from build123d import *

# Parameters (mm, degrees)
SKETCH_W       = 31.75
SKETCH_H       = 31.75
SKETCH_W_2     = 26.2128
SKETCH_H_2     = 26.2128
PAD_DEPTH      = 152.4
PAD_DEPTH_BACK = 152.4
POCKET_DEPTH   = 31.75


with BuildPart() as part:
    # Sketch → Pad (new body, two sides)
    with BuildSketch(Plane.YZ) as pad_sk:
        Rectangle(SKETCH_W, SKETCH_H)
        Rectangle(SKETCH_W_2, SKETCH_H_2, mode=Mode.SUBTRACT)
    extrude(amount=PAD_DEPTH)
    extrude(pad_sk.sketch, amount=-PAD_DEPTH_BACK)

    # Sketch001 → Pocket (cut)
    with BuildSketch(Plane(origin=(0, 0, 15.875), x_dir=(0, -1, 0), z_dir=(0, 0, 1))):
        Polygon((15.875, 152.4), (-15.875, 152.4), (-15.875, 120.65), align=None)
    pocket = extrude(amount=-POCKET_DEPTH, mode=Mode.SUBTRACT)

    # Mirrored: Pocket across Sketch001 H_Axis
    add(pocket.mirror(Plane(origin=(0, 0, 15.875), x_dir=(0, 0, 1), z_dir=(1, 0, 0))), mode=Mode.SUBTRACT)


solid = part.part
Model file for the job. Use its own axes, mm. A direction names the side the tool comes from. Give positions to 0.01 mm unless a question says otherwise; leave off trailing zeros. Order: outer loops, then holes, each group sorted by start corner. A loop starts at its lowest first (then second) coordinate and runs counter-clockwise, first axis right, second up. Notation, with made-up numbers: (33, -36.75) - (60, -36.75) arc R20 cw to (60, -9.75) - close; hole circle Ø4 at (82.25, 54.5). An arc over 180 degrees is marked (long way). One line per item, written item: value.
Item 1: Two-plate mould, pull along Z, no slides. Class faces 3 (the flat face through (2, 0, -15.875)), 4 (the flat face through (136.303, 0.222, -13.889)), 5 (the flat face through (2, 0, -13.106)): released by +Z, released by -Z, zero draft, split by the parting line, or undercut.
Response values:
face 3: released by -Z
face 4: zero draft
face 5: undercut
Item 2: Pin check, flat tips, straight feed: pin 1 Ø10 at (y, z) = (-10, -7) entering from -X (3 decimals); pin 2 Ø6 at (y, z) = (5.5, 12.5) entering from -X; pin 3 Ø8 at (y, z) = (7, -5.5) entering from -X. Stop position of each tip, or through.
Response values:
pin 1: x = -151.525
pin 2: x = -133.96
pin 3: through
Item 3: Slice it at A-A (z = 1). List the corners of the cut face in (x, y) (3 decimals).
Response values:
outline: (-152.4, -15.875) - (152.4, -15.875) - (149.631, -13.106) - (-149.631, -13.106) - close; (-123.419, 13.106) - (123.419, 13.106) - (120.65, 15.875) - (-120.65, 15.875) - close
Item 4: Slice it at D-D (x = -129.5). List the corners of the cut face in (y, z) (3 decimals), then the cut area to 3 significant figures.
Response values:
outline: (-15.875, -15.875) - (7.025, -15.875) - (7.025, -13.106) - (-13.106, -13.106) - (-13.106, 13.106) - (7.025, 13.106) - (7.025, 15.875) - (-15.875, 15.875) - close
area: 199 mm2
Item 5: Slice it at B-B (x = 96.5). List the corners of the cut face in (y, z) (3 decimals), then the cut area to 3 significant figures.
Response values:
outline: (-15.875, -15.875) - (15.875, -15.875) - (15.875, 15.875) - (-15.875, 15.875) - close; hole (-13.106, -13.106) - (13.106, -13.106) - (13.106, 13.106) - (-13.106, 13.106) - close
area: 321 mm2
Item 6: Tool access for faces 1 (the flat face through (2, 15.875, 0)), 2 (the flat face through (2, 13.106, 0)): list every direction of +Z, -Z, +X, -X, +Y, -Y with a clear straight run to the whole face (end or side of a thin tool).
Response values:
face 1: +Z, -Z, +X, -X, +Y
face 2: +X, -X
Item 7: Wall check: line 1 (Y direction, x = 23, z = 8) (3 decimals); line 2 (Y direction, x = -123, z = -10) (3 decimals). Give the ranges that are in metal, low to high.
Response values:
line 1: -15.875 to -13.106, 13.106 to 15.875
line 2: -15.875 to -13.106, 13.106 to 13.525
Item 8: Slice it at C-C (y = -0.5). List the corners of the cut face in (x, z) (3 decimals), then the cut area to 3 significant figures.
Response values:
outline: (-137.025, -15.875) - (137.025, -15.875) - (137.025, -13.106) - (-137.025, -13.106) - close; (-137.025, 13.106) - (137.025, 13.106) - (137.025, 15.875) - (-137.025, 15.875) - close
area: 1,520 mm2
